Geometry: final body of the model. Coordinates: model frame, mm. A direction names the side the tool comes from. Give positions to 0.01 mm unless a question says otherwise; leave off trailing zeros. Write each loop counter-clockwise with the first axis right and the second up, starting at its lowest first coordinate (ties: lowest second). Pieces come first, ordered by that corner, then holes. Notation, with made-up numbers: M 17,18.25 L 59,18.25 A28 cw 59,44.25 Z; hole C 36,-9 d3. An arc over 180 degrees is marked long. One line per question, with ' | ' between items.
from build123d import *

# Parameters (mm, degrees)
CROQUIS1_W              = 60
CROQUIS1_H              = 50
SALIENTE_EXTRUIR1_DEPTH = 12.75
CORTAR_EXTRUIR2_START   = 12.75
CROQUIS2_W              = 55
CROQUIS2_H              = 45
CORTAR_EXTRUIR2_DEPTH   = 10.25
CROQUIS3_W              = 4
CROQUIS3_H              = 6.5
CORTAR_EXTRUIR3_DEPTH   = 10.25
CROQUIS5_W              = 49
CROQUIS5_H              = 7.25
CORTAR_EXTRUIR4_DEPTH   = 45.125
CROQUIS6_W              = 7.5
CROQUIS6_H              = 4
CROQUIS6_W_2            = 12.5
CORTAR_EXTRUIR5_DEPTH   = 60
CROQUIS8_W              = 7.141428429
CROQUIS8_H              = 7
SALIENTE_EXTRUIR6_DEPTH = 5.5


with BuildPart() as part:
    # Croquis1 → Saliente-Extruir1 (new body)
    with BuildSketch(Plane(origin=(0, 0, 0), x_dir=(1, 0, 0), z_dir=(0, 1, 0))):
        Rectangle(CROQUIS1_W, CROQUIS1_H)
    extrude(amount=SALIENTE_EXTRUIR1_DEPTH)

    # Croquis2 → Cortar-Extruir2 (cut)
    with BuildSketch(Plane(origin=(0, 0, 0), x_dir=(1, 0, 0), z_dir=(0, 1, 0)).offset(CORTAR_EXTRUIR2_START)):
        Rectangle(CROQUIS2_W, CROQUIS2_H)
    extrude(amount=-CORTAR_EXTRUIR2_DEPTH, mode=Mode.SUBTRACT)

    # Croquis3 → Cortar-Extruir3 (cut)
    with BuildSketch(Plane(origin=(0, 0, 0), x_dir=(1, 0, 0), z_dir=(0, 1, 0))):
        with Locations((-1, -7)):
            Rectangle(CROQUIS3_W, CROQUIS3_H)
    extrude(amount=CORTAR_EXTRUIR3_DEPTH, mode=Mode.SUBTRACT)

    # Croquis5 → Cortar-Extruir4 (cut, symmetric)
    with BuildSketch(Plane.XY):
        with Locations((0, 9.125)):
            Rectangle(CROQUIS5_W, CROQUIS5_H)
    extrude(amount=CORTAR_EXTRUIR4_DEPTH, both=True, mode=Mode.SUBTRACT)

    # Croquis6 → Cortar-Extruir5 (cut)
    with BuildSketch(Plane(origin=(0, 0, 0), x_dir=(0, 0, -1), z_dir=(1, 0, 0))):
        with Locations((-10.75, 9.25)):
            Rectangle(CROQUIS6_W, CROQUIS6_H)
        with Locations((13.25, 9.25)):
            Rectangle(CROQUIS6_W_2, CROQUIS6_H)
    extrude(amount=CORTAR_EXTRUIR5_DEPTH, mode=Mode.SUBTRACT)

    # Croquis8 → Saliente-Extruir6 (add)
    with BuildSketch(Plane(origin=(0, 0, 0), x_dir=(1, 0, 0), z_dir=(0, 1, 0))):
        with Locations((23.929285785, -19)):
            Rectangle(CROQUIS8_W, CROQUIS8_H)
        with Locations((-23.929285785, -19)):
            Rectangle(CROQUIS8_W, CROQUIS8_H)
        with Locations((23.929285785, 19)):
            Rectangle(CROQUIS8_W, CROQUIS8_H)
        with Locations((-23.929285785, 19)):
            Rectangle(CROQUIS8_W, CROQUIS8_H)
    extrude(amount=SALIENTE_EXTRUIR6_DEPTH)


solid = part.part
(1) Draft query along X for faces 1 (the face through (-30, 6, 0)), 2 (the face through (0, 5.5, -23)), 3 (the face through (-29, 12.75, 0)). Return one class per face: released by +X, released by -X, zero draft, split by the parting line, or undercut.
Working result:
face 1: released by -X | face 2: undercut | face 3: zero draft
(2) Cut plane B-B, the plane z = -18. Return loops of the section in (x, y).
Working result:
outline: M -30,0 L 30,0 L 30,7.25 L 27.5,7.25 L 27.5,5.5 L 20.36,5.5 L 20.36,2.5 L -20.36,2.5 L -20.36,5.5 L -27.5,5.5 L -27.5,12.75 L -30,12.75 Z; M 27.5,11.25 L 30,11.25 L 30,12.75 L 27.5,12.75 Z
(3) Set-up query: faces 4 (the face through (20.359, 4, -19)), 5 (the face through (1, 1, 7)), 6 (the face through (29, 7.25, 11)). Return all of +Z, -Z, +X, -X, +Y, -Y with unobstructed straight access to the full face (end or side cutting, diameter ignored); none if empty.
Working result:
face 4: +Y | face 5: +Y, -Y | face 6: +X
(4) Cut plane A-A, the plane y = 9.25. Return loops of the section in (x, z), then the cut area to 3 significant figures.
Working result:
outline: M -30,-25 L -24.5,-25 L -24.5,-22.5 L -27.5,-22.5 L -27.5,22.5 L -24.5,22.5 L -24.5,25 L -30,25 Z; M 24.5,-25 L 30,-25 L 30,-19.5 L 27.5,-19.5 L 27.5,-22.5 L 24.5,-22.5 Z; M 24.5,22.5 L 27.5,22.5 L 27.5,14.5 L 30,14.5 L 30,25 L 24.5,25 Z; M 27.5,-7 L 30,-7 L 30,7 L 27.5,7 Z | area: 230 mm^2
(5) First-contact query: P1, Ø8, axis at x = 7, z = -12, coming from the +Y side. Flat tip, straight axial feed; report the tip coordinate or a pass-through.
Working result:
P1: stops at y = 2.5
(6) Cut plane C-C, the plane x = 21.5. Return loops of the section in (y, z), then the cut area to 3 significant figures.
Working result:
outline: M 0,-25 L 5.5,-25 L 5.5,-15.5 L 2.5,-15.5 L 2.5,15.5 L 5.5,15.5 L 5.5,25 L 0,25 Z | area: 182 mm^2
(7) Cut plane D-D, the plane z = 1.5. Return loops of the section in (x, y).
Working result:
outline: M -30,0 L 30,0 L 30,12.75 L 27.5,12.75 L 27.5,2.5 L -27.5,2.5 L -27.5,12.75 L -30,12.75 Z
(8) Material intervals for L1, parallel to X at y = 7.25, z = -21.5; L2, parallel to Z at x = 10.5, y = 4.75; L3, parallel to Y at x = -16, z = -20, sorted ascending. Write a range as [from, to].
Working result:
L1: x = [-30, -27.5], [27.5, 30] | L2: z = [-25, -22.5], [22.5, 25] | L3: y = [0, 2.5]
